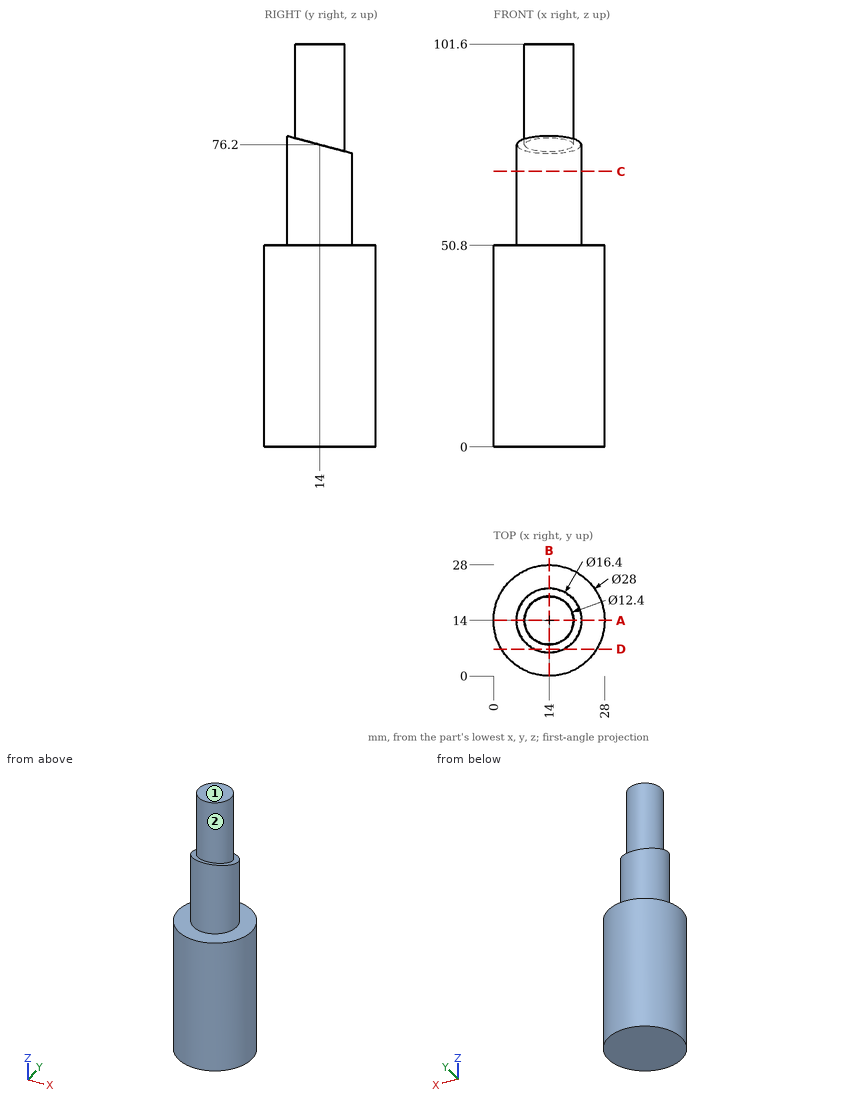
Job drawing, mm, ordinate dimensions from the low corner. One solid piece. A direction names the side the tool comes from. Coordinates: 2 decimals unless noted, no trailing zeros. Write each loop counter-clockwise with the first axis right and the second up, starting at its lowest first coordinate (ties: lowest second). Pieces come first, ordered by that corner, then holes. Notation, with made-up numbers: (17.25, -28) - (61.25, -28) arc R28 cw to (61.25, -6) - close; hole circle Ø5 at (-33, 73.5). An arc over 180 degrees is marked (long way). Use a Markdown table: item, result. Add a question column.
Item 1: Band-saw the part on A-A, the plane y = 14. Give the cut face in (x, z).
Item 2: Band-saw the part on B-B, the plane x = 14. Give the cut face in (y, z).
Item 3: Drill centre lines: L1, parallel to Z at x = 3, y = 10.5; L2, parallel to X at y = 14.5, z = 37; L3, parallel to X at y = 13.5, z = 53.5. Where is each one in solid material? Low to high. Write a range as from..to.
Item 4: 3-axis set-ups, long thin cutter, end or side, ignore diameter. For the marked faces 1 and 2: which of +Z, -Z, +X, -X, +Y, -Y reach the whole face in a straight line?
Item 5: Band-saw the part on D-D, the plane y = 6.75. Give the cut face in (x, z), and give its area (3 significant figures).
Item 6: Band-saw the part on C-C, the plane z = 69.5. Give the cut face in (x, y).
Item 7: Flat gauge pins, fed straight in: pin 1 (4 mm diameter, centred on x = 6.5, z = 59, fed in from -Y); pin 2 (12 mm diameter, centred on y = 14, z = 87.5, fed in from -X); pin 3 (1.5 mm diameter, centred on x = 8, z = 67.5, fed in from +Y). Where does each tip first touch, or does it go through?
Numbers:
| question | item | result |
|---|---|---|
| 1 | outline | (0, 0) - (28, 0) - (28, 50.8) - (22.2, 50.8) - (22.2, 76.2) - (20.2, 76.2) - (20.2, 101.6) - (7.8, 101.6) - (7.8, 76.2) - (5.8, 76.2) - (5.8, 50.8) - (0, 50.8) - close |
| 2 | outline | (0, 0) - (28, 0) - (28, 50.8) - (22.2, 50.8) - (22.2, 74) - (20.2, 74.54) - (20.2, 101.6) - (7.8, 101.6) - (7.8, 77.86) - (5.8, 78.4) - (5.8, 50.8) - (0, 50.8) - close |
| 3 | L1 | 0..50.8 |
| 3 | L2 | 0.01..27.99 |
| 3 | L3 | 5.82..22.18 |
| 4 | face 1 | +Z, +X, -X, +Y, -Y |
| 4 | face 2 | +Z |
| 5 | outline | (2.02, 0) - (25.98, 0) - (25.98, 50.8) - (17.83, 50.8) - (17.83, 78.14) - (10.17, 78.14) - (10.17, 50.8) - (2.02, 50.8) - close |
| 5 | area | 1,430 mm2 |
| 6 | outline | circle Ø16.4 at (14, 14) |
| 7 | pin 1 | y = 7.92 |
| 7 | pin 2 | x = 7.8 |
| 7 | pin 3 | y = 20.3 |
